Work out the finished part from the listing and answer in its coordinate system (mm). A direction names the side the tool comes from. Give positions to 0.01 mm unless a question says otherwise; leave off trailing zeros. Loops run counter-clockwise (first coordinate to the right, second up) from the corner with the lowest first, then second, coordinate; pieces in that order, holes last. Notation, with made-up numbers: M 51,32.5 L 96,32.5 A12 cw 96,36.5 Z; hole C 71,-8 d8. An arc over 180 degrees is marked long. Write item = value, one per line. Start each with the question number.
1. The mould has two halves that part along Z. Classify faces 1 (the face through (61.71, -3.94, 49.68)), 2 (the face through (0, -9, 108)), 3 (the face through (44, -9, 220)): released by +Z, released by -Z, zero draft, split by the parting line, or undercut.
2. Consider L1, parallel to Z at x = 45, y = -4 (3 decimals); L2, parallel to Z at x = 49, y = -17.5; L3, parallel to X at y = -15, z = 211. Determine where each line is inside the solid, lowest interval first. Write a range as [from, to].
3. For faces 4 (the face through (71.19, -17.52, 192.05)), 5 (the face through (20, -8, 36)), 6 (the face through (64.36, -5.42, 8.7)), determine the directions among +Z, -Z, +X, -X, +Y, -Y from which every point of the face is accessible in a straight line to the end or side of a thin tool.
4. Section C-C on z = 210 is taken. Determine the outline of the cut face in (x, y) (3 decimals), plus the area to 3 significant figures.
5. Section A-A on x = 45 is taken. Determine the outline of the cut face in (y, z) (3 decimals), plus the area to 3 significant figures.
6. Section D-D on z = 166.5 is taken. Determine the outline of the cut face in (x, y).
7. Section B-B on y = -3.75 is taken. Give the number of separate pieces and of enclosed holes in the cut face, plus the area to 3 significant figures.
8. Flat-ended cylindrical pins translate along their axes: pin 1 Ø5 at (x, z) = (69, 190) entering from -Y; pin 2 Ø5.5 at (x, z) = (65, 56) entering from +Y; pin 3 Ø9 at (x, z) = (22.5, 210) entering from -Y. Find the tip coordinate at first contact, or state that the pin passes through.
```python
from build123d import *

# Parameters (mm, degrees)
F0_W           = 90
F0_H           = 220
F1_DEPTH       = 19
F3_D           = 6.8
F3_CBORE_D     = 14.25
F3_CBORE_DEPTH = 8
F5_DEPTH       = 3
F7_D           = 11
F7_CBORE_D     = 17.25
F7_CBORE_DEPTH = 10
F9_D           = 8.8
F9_CBORE_D     = 14.25
F9_CBORE_DEPTH = 8


with BuildPart() as f1:
    # F0 (on Front) → F1 (new body)
    with BuildSketch(Plane.XZ):
        with Locations((45, 110)):
            Rectangle(F0_W, F0_H)
    extrude(amount=F1_DEPTH)

    # F3 (through all)
    with Locations(Plane.XZ.offset(19)):
        with Locations((22.5, 210), (67.5, 210), (22.5, 10), (67.5, 10)):
            CounterBoreHole(F3_D / 2, F3_CBORE_D / 2, F3_CBORE_DEPTH)

    # F4 (on face) → F5 (cut)
    with BuildSketch(Plane.XZ.offset(19)):
        with BuildLine():
            ThreePointArc((24, 190), (18.8786796564, 192.1213203436), (21, 187))
            Line((21, 187), (21, 103))
            ThreePointArc((21, 103), (18.8786796564, 97.8786796564), (24, 100))
            Line((24, 100), (66, 100))
            ThreePointArc((66, 100), (71.1213203436, 97.8786796564), (69, 103))
            Line((69, 103), (69, 187))
            ThreePointArc((69, 187), (71.1213203436, 192.1213203436), (66, 190))
            Line((66, 190), (24, 190))
        make_face()
    extrude(amount=-F5_DEPTH, mode=Mode.SUBTRACT)

    # F7 (through all)
    with Locations(Plane(origin=(0, 0, 0), x_dir=(-1, 0, 0), z_dir=(0, 1, 0))):
        with Locations((-45, 170), (-45, 115)):
            CounterBoreHole(F7_D / 2, F7_CBORE_D / 2, F7_CBORE_DEPTH)

    # F9 (through all)
    with Locations(Plane(origin=(0, 0, 0), x_dir=(-1, 0, 0), z_dir=(0, 1, 0))):
        with Locations((-65, 56), (-25, 36)):
            CounterBoreHole(F9_D / 2, F9_CBORE_D / 2, F9_CBORE_DEPTH)


solid = f1.part
```
Verdict:
q1.face_1 = undercut
q1.face_2 = zero draft
q1.face_3 = released by +Z
q2.L1 = [0, 106.375], [123.625, 161.375], [178.625, 220]
q2.L2 = [0, 100], [190, 220]
q2.L3 = [0, 15.45], [29.55, 60.45], [74.55, 90]
q3.face_4 = -Y
q3.face_5 = +Y
q3.face_6 = +Y, -Y
q4.outline = M 0,-19 L 15.375,-19 L 15.375,-11 L 19.1,-11 L 19.1,0 L 0,0 Z; M 25.9,-11 L 29.625,-11 L 29.625,-19 L 60.375,-19 L 60.375,-11 L 64.1,-11 L 64.1,0 L 25.9,0 Z; M 70.9,-11 L 74.625,-11 L 74.625,-19 L 90,-19 L 90,0 L 70.9,0 Z
q4.area = 1,330 mm2
q5.outline = M -19,0 L 0,0 L 0,106.375 L -10,106.375 L -10,109.5 L -16,109.5 L -16,100 L -19,100 Z; M -19,190 L -16,190 L -16,175.5 L -10,175.5 L -10,178.625 L 0,178.625 L 0,220 L -19,220 Z; M -16,120.5 L -10,120.5 L -10,123.625 L 0,123.625 L 0,161.375 L -10,161.375 L -10,164.5 L -16,164.5 Z
q5.area = 3,430 mm2
q6.outline = M 0,-19 L 21,-19 L 21,-16 L 40.76,-16 L 40.76,-10 L 37.12,-10 L 37.12,0 L 0,0 Z; M 49.24,-16 L 69,-16 L 69,-19 L 90,-19 L 90,0 L 52.88,0 L 52.88,-10 L 49.24,-10 Z
q7.separate_pieces = 1
q7.enclosed_holes = 8
q7.area = 18,900 mm2
q8.pin_1 = -16
q8.pin_2 = through
q8.pin_3 = -11
